from build123d import *

# Parameters (mm, degrees)
F0_W     = 80
F0_H     = 90
F1_DEPTH = 8
F3_DEPTH = 82
F4_DEPTH = 77
F5_DEPTH = 70
F6_DEPTH = 68
F7_DEPTH = 62
F8_DEPTH = 5


with BuildPart() as f1:
    # F0 (on Top) → F1 (new body)
    with BuildSketch(Plane.XY):
        with Locations((-20.8165652305, -23.7756354961)):
            Rectangle(F0_W, F0_H)
    extrude(amount=F1_DEPTH)

    # F2 (on face) → F3 (cut)
    with BuildSketch(Plane.XZ.offset(68.7756354961)):
        with BuildLine():
            ThreePointArc((-57.8165652305, 8), (-53.8165652305, 4), (-49.8165652305, 8))
            Line((-49.8165652305, 8), (-57.8165652305, 8))
        make_face()
        with BuildLine():
            Line((-39.8165652305, 8), (-47.8165652305, 8))
            ThreePointArc((-47.8165652305, 8), (-43.8165652305, 4), (-39.8165652305, 8))
        make_face()
    extrude(amount=-F3_DEPTH, mode=Mode.SUBTRACT)

    # F2 (on face) → F4 (cut)
    with BuildSketch(Plane.XZ.offset(68.7756354961)):
        with BuildLine():
            Line((-31.8165652305, 8), (-37.8165652305, 8))
            ThreePointArc((-37.8165652305, 8), (-34.8165652305, 5), (-31.8165652305, 8))
        make_face()
        with BuildLine():
            Line((-23.8165652305, 8), (-29.8165652305, 8))
            ThreePointArc((-29.8165652305, 8), (-26.8165652305, 5), (-23.8165652305, 8))
        make_face()
    extrude(amount=-F4_DEPTH, mode=Mode.SUBTRACT)

    # F2 (on face) → F5 (cut)
    with BuildSketch(Plane.XZ.offset(68.7756354961)):
        with BuildLine():
            Line((-16.8165652305, 8), (-21.8165652305, 8))
            ThreePointArc((-21.8165652305, 8), (-19.3165652305, 5.5), (-16.8165652305, 8))
        make_face()
        with BuildLine():
            Line((-9.8165652305, 8), (-14.8165652305, 8))
            ThreePointArc((-14.8165652305, 8), (-12.3165652305, 5.5), (-9.8165652305, 8))
        make_face()
    extrude(amount=-F5_DEPTH, mode=Mode.SUBTRACT)

    # F2 (on face) → F6 (cut)
    with BuildSketch(Plane.XZ.offset(68.7756354961)):
        with BuildLine():
            Line((-3.7165652305, 8), (-7.8165652305, 8))
            ThreePointArc((-7.8165652305, 8), (-5.7665652305, 5.95), (-3.7165652305, 8))
        make_face()
        with BuildLine():
            ThreePointArc((-1.7165652305, 8), (0.3334347695, 5.95), (2.3834347695, 8))
            Line((2.3834347695, 8), (-1.7165652305, 8))
        make_face()
    extrude(amount=-F6_DEPTH, mode=Mode.SUBTRACT)

    # F2 (on face) → F7 (cut)
    with BuildSketch(Plane.XZ.offset(68.7756354961)):
        with BuildLine():
            ThreePointArc((4.3834347695, 8), (6.4334347695, 5.95), (8.4834347695, 8))
            Line((8.4834347695, 8), (4.3834347695, 8))
        make_face()
        with BuildLine():
            ThreePointArc((10.4834347695, 8), (12.5334347695, 5.95), (14.5834347695, 8))
            Line((14.5834347695, 8), (10.4834347695, 8))
        make_face()
    extrude(amount=-F7_DEPTH, mode=Mode.SUBTRACT)

    # F2 (on face) → F8 (join)
    with BuildSketch(Plane.XZ.offset(68.7756354961)):
        with BuildLine():
            ThreePointArc((-57.8165652305, 8), (-53.8165652305, 4), (-49.8165652305, 8))
            Line((-49.8165652305, 8), (-57.8165652305, 8))
        make_face()
        with BuildLine():
            Line((-39.8165652305, 8), (-47.8165652305, 8))
            ThreePointArc((-47.8165652305, 8), (-43.8165652305, 4), (-39.8165652305, 8))
        make_face()
        with BuildLine():
            Line((-31.8165652305, 8), (-37.8165652305, 8))
            ThreePointArc((-37.8165652305, 8), (-34.8165652305, 5), (-31.8165652305, 8))
        make_face()
        with BuildLine():
            Line((-23.8165652305, 8), (-29.8165652305, 8))
            ThreePointArc((-29.8165652305, 8), (-26.8165652305, 5), (-23.8165652305, 8))
        make_face()
        with BuildLine():
            Line((-16.8165652305, 8), (-21.8165652305, 8))
            ThreePointArc((-21.8165652305, 8), (-19.3165652305, 5.5), (-16.8165652305, 8))
        make_face()
        with BuildLine():
            Line((-9.8165652305, 8), (-14.8165652305, 8))
            ThreePointArc((-14.8165652305, 8), (-12.3165652305, 5.5), (-9.8165652305, 8))
        make_face()
        with BuildLine():
            Line((-3.7165652305, 8), (-7.8165652305, 8))
            ThreePointArc((-7.8165652305, 8), (-5.7665652305, 5.95), (-3.7165652305, 8))
        make_face()
        with BuildLine():
            ThreePointArc((-1.7165652305, 8), (0.3334347695, 5.95), (2.3834347695, 8))
            Line((2.3834347695, 8), (-1.7165652305, 8))
        make_face()
        with BuildLine():
            ThreePointArc((4.3834347695, 8), (6.4334347695, 5.95), (8.4834347695, 8))
            Line((8.4834347695, 8), (4.3834347695, 8))
        make_face()
        with BuildLine():
            ThreePointArc((10.4834347695, 8), (12.5334347695, 5.95), (14.5834347695, 8))
            Line((14.5834347695, 8), (10.4834347695, 8))
        make_face()
    extrude(amount=-F8_DEPTH)


solid = f1.part
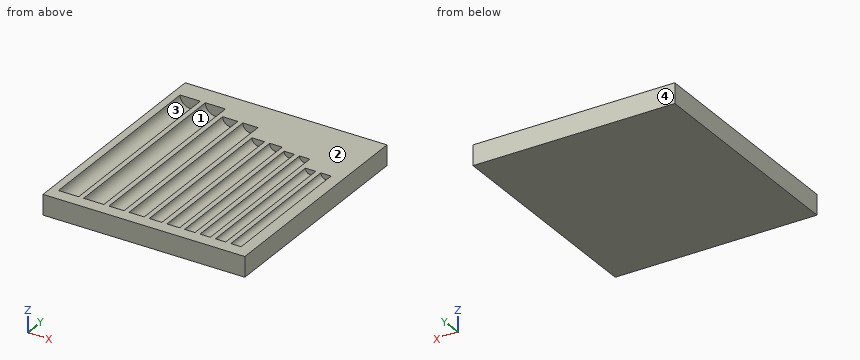
Check sheet for the modelled part. Datum: model origin and axes. Units: mm. Face numbers are marked on the shaded views. Give positions to 0.01 mm unless a question says otherwise; leave off trailing zeros. Loops run counter-clockwise (first coordinate to the right, second up) from the corner with the lowest first, then second, coordinate; pieces in that order, holes last. Notation, with made-up numbers: M 80.25,86 L 93.25,86 A31 ccw 93.25,113 Z; hole C 76,-31 d3. An arc over 180 degrees is marked long. Use a Markdown table: item, result. Add a question column.
Q1. Sectioned sample at C-C, the plane x = 7.5. Record the cut outline in (y, z).
Q2. Sectioned sample at A-A, the plane y = -61.5. Record the cut outline in (x, z).
Q3. Sectioned sample at B-B, the plane x = -27.5. Record the cut outline in (y, z), then the cut area to 3 significant figures.
Q4. Mould release check, pull along Y, two halves, no side actions. Record for the marked faces 1, 2, 3 and 4: pulls with the +Y half, pulls with the -Y half, needs draft (parallel to the pull), parting line crosses it, or undercut.
Q5. Scan lines: line 1 along Y through (x, z) = (-51, 6.25); line 2 along Z through (x, y) = (0.5, -43.5); line 3 along X through (y, z) = (8, 7) (3 decimals). Record each from-to range of solid material in increasing order. Write a range as [from, to].
Verdict:
| question | item | result |
|---|---|---|
| 1 | outline | M -68.78,0 L 21.22,0 L 21.22,8 L -6.78,8 L -6.78,6.25 L -63.78,6.25 L -63.78,8 L -68.78,8 Z |
| 2 | outline | M -60.82,0 L 19.18,0 L 19.18,8 L 14.58,8 A2.05 cw 10.48,8 L 8.48,8 A2.05 cw 4.38,8 L 2.38,8 A2.05 cw -1.72,8 L -3.72,8 A2.05 cw -7.82,8 L -9.82,8 A2.5 cw -14.82,8 L -16.82,8 A2.5 cw -21.82,8 L -23.82,8 A3 cw -29.82,8 L -31.82,8 A3 cw -37.82,8 L -39.82,8 A4 cw -47.82,8 L -49.82,8 A4 cw -57.82,8 L -60.82,8 Z |
| 3 | outline | M -68.78,0 L 21.22,0 L 21.22,8 L 8.22,8 L 8.22,5.08 L -63.78,5.08 L -63.78,8 L -68.78,8 Z |
| 3 | area | 510 mm^2 |
| 4 | face 1 | undercut |
| 4 | face 2 | needs draft |
| 4 | face 3 | undercut |
| 4 | face 4 | pulls with the +Y half |
| 5 | line 1 | [-68.78, -63.78], [13.22, 21.22] |
| 5 | line 2 | [0, 5.96] |
| 5 | line 3 | [-60.817, -57.69], [-49.944, -47.69], [-39.944, -37.645], [-31.988, -29.645], [-23.988, 19.183] |
